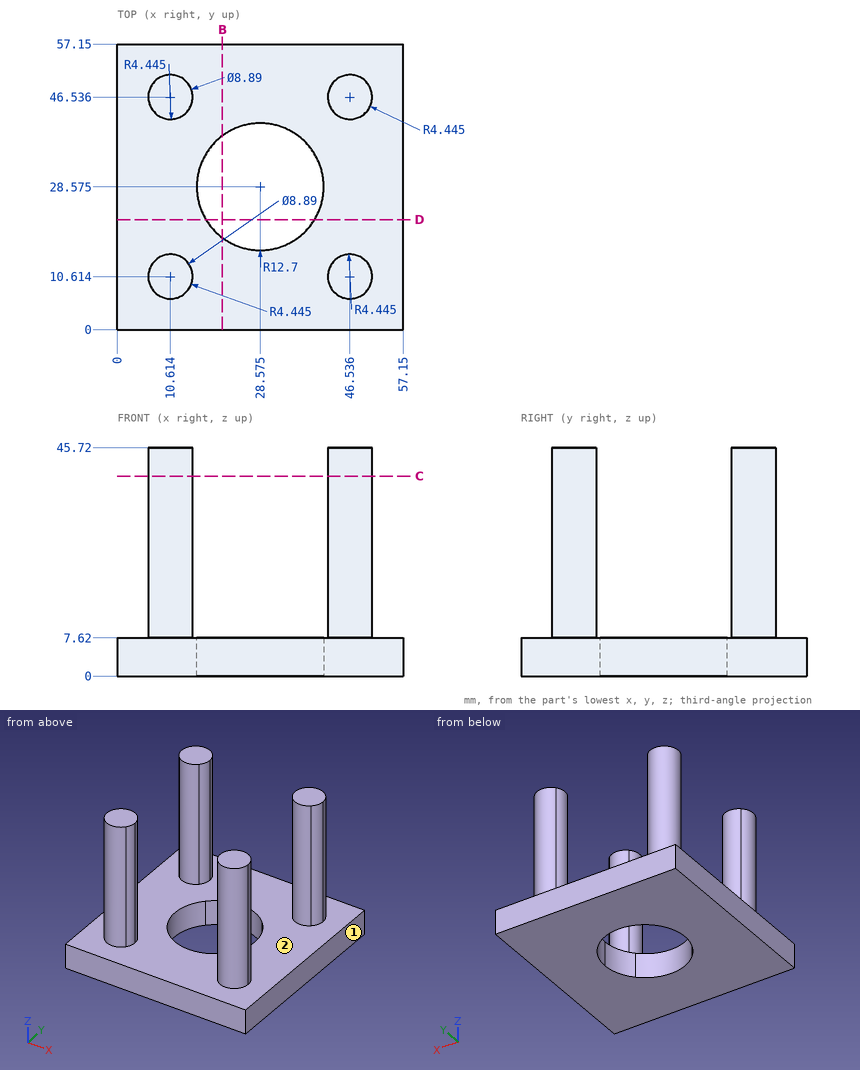
Could you check a few things on this drawing? It's one solid part, dimensions in mm from its lowest x, y, z. A direction names the side the tool comes from. Coordinates: 2 decimals unless noted, no trailing zeros. Write each loop counter-clockwise with the first axis right and the second up, starting at its lowest first coordinate (ties: lowest second). Pieces come first, ordered by that corner, then holes.
1) If we section it at B-B (x = 21): List the corners of the cut face in (y, z) for me, plus the area to 3 significant figures.
Filled in:
outline: (0, 0) - (18.38, 0) - (18.38, 7.62) - (0, 7.62) - close; (38.77, 0) - (57.15, 0) - (57.15, 7.62) - (38.77, 7.62) - close
area: 280 mm2
2) Which directions (+Z, -Z, +X, -X, +Y, -Y) give clear straight access to the entire face, cutting with the end or side of a thin tool? Please do the marked faces 1 and 2.
Filled in:
face 1: +Z, -Z, +X, +Y, -Y
face 2: +Z
3) If we section it at D-D (y = 22): List the corners of the cut face in (x, z) for me, plus the area to 3 significant figures.
Filled in:
outline: (0, 0) - (17.71, 0) - (17.71, 7.62) - (0, 7.62) - close; (39.44, 0) - (57.15, 0) - (57.15, 7.62) - (39.44, 7.62) - close
area: 270 mm2
4) I'm going to push flat-ended pins straight in: pin 1 (5 mm diameter, centred on x = 19.5, y = 24, fed in from +Z); pin 2 (1.5 mm diameter, centred on y = 10, z = 26.5, fed in from -X); pin 3 (1 mm diameter, centred on y = 44, z = 12.5, fed in from -X); pin 4 (3 mm diameter, centred on x = 43, z = 38, fed in from +Y). Where does each tip first touch, or does it pass through?
Filled in:
pin 1: passes through
pin 2: stops at x = 6.17
pin 3: stops at x = 6.66
pin 4: stops at y = 50.49
5) If I drill on line 1 (X direction, y = 46.5, z = 9); line 2 (X direction, y = 50, z = 25); line 3 (Z direction, x = 50, y = 7.5), over which ranges is the centre line in solid material (lowest first)?
Filled in:
line 1: x = 6.17 to 15.06, 42.09 to 50.98
line 2: x = 7.83 to 13.4, 43.75 to 49.32
line 3: z = 0 to 7.62
6) If we section it at C-C (z = 40): List the corners of the cut face in (x, y) for me (1 decimal).
Filled in:
outline: circle Ø8.9 at (10.6, 10.6); circle Ø8.9 at (10.6, 46.5); circle Ø8.9 at (46.5, 10.6); circle Ø8.9 at (46.5, 46.5)
